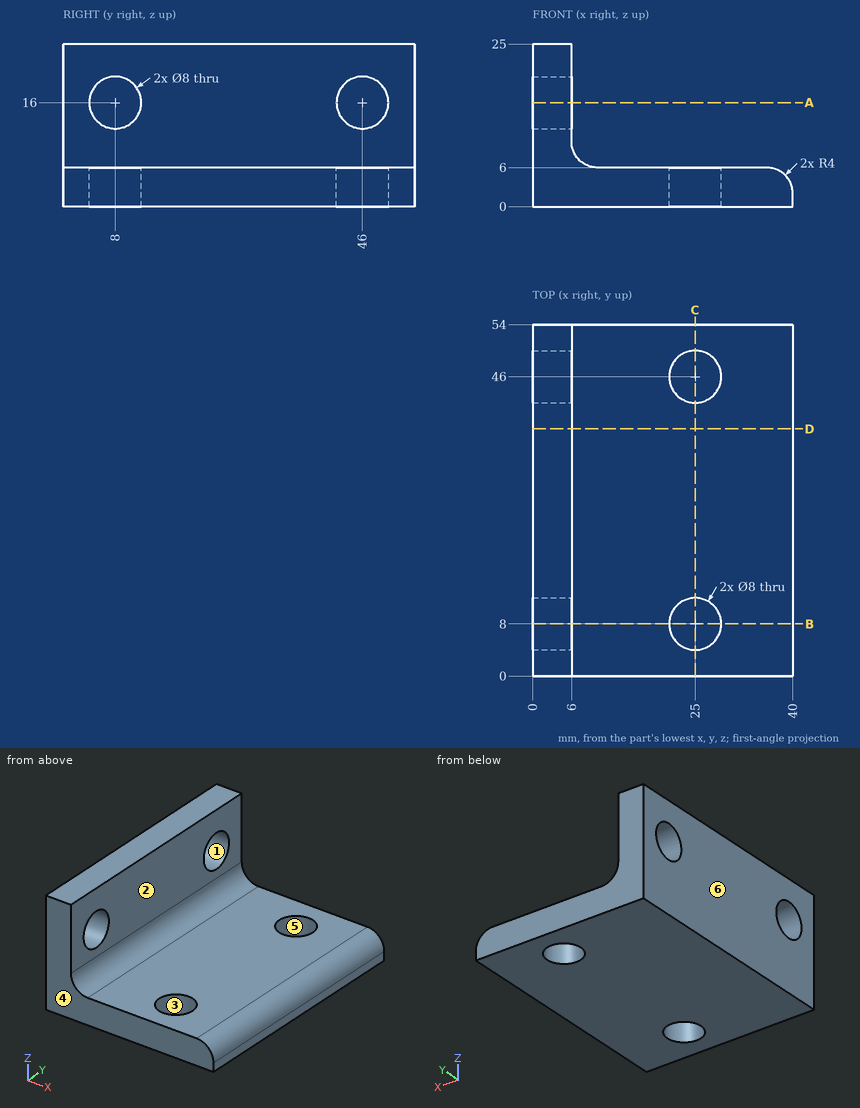
Input: dimensioned drawing with shaded views. Units: mm. Origin: part minimum x, y, z. A direction names the side the tool comes from. Give positions to 0.01 mm unless a question says otherwise; leave off trailing zeros. Write each loop counter-clockwise with the first axis right and the second up, starting at its lowest first coordinate (ties: lowest second). Pieces come first, ordered by that corner, then holes. Notation, with made-up numbers: (62.5, -27) - (92.5, -27) arc R23 ccw to (92.5, -15) - close; hole circle Ø4 at (-12.5, 86). An arc over 180 degrees is marked (long way). Write item = value, one per line. Start each with the question number.
1) Cut plane A-A (z = 16). Return loops of the section in (x, y), and give its area (3 significant figures).
2) Cut plane C-C (x = 25). Return loops of the section in (y, z), and give its area (3 significant figures).
3) Material intervals for L1, parallel to X at y = 8, z = 2.1; L2, parallel to Y at x = 2, z = 12.5; L3, parallel to Z at x = 1.7, y = 46, sorted ascending. Write a range as [from, to].
4) Pin query (flat end, axial travel): pin 1 (4 mm diameter, centred on x = 23.5, y = 16, fed in from -Z); pin 2 (7.5 mm diameter, centred on y = 23, z = 21, fed in from +X); pin 3 (6 mm diameter, centred on x = 30, y = 23.5, fed in from +Z). Return the tip coordinate at first contact, or that it passes through.
5) Reachability of the marked faces 1 and 2 from +Z, -Z, +X, -X, +Y, -Y: full face, straight path, thin tool, end or side. Return the list, or none.
6) Draft query along X for the marked faces 3, 4, 5 and 6. Return one class per face: pulls with the +X half, pulls with the -X half, needs draft (parallel to the pull), parting line crosses it, or undercut.
7) Cut plane D-D (y = 38). Return loops of the section in (x, z).
8) Cut plane B-B (y = 8). Return loops of the section in (x, z).
Answers follow:
q1.outline = (0, 0) - (6, 0) - (6, 4) - (0, 4) - close; (0, 12) - (6, 12) - (6, 42) - (0, 42) - close; (0, 50) - (6, 50) - (6, 54) - (0, 54) - close
q1.area = 228 mm^2
q2.outline = (0, 0) - (4, 0) - (4, 6) - (0, 6) - close; (12, 0) - (42, 0) - (42, 6) - (12, 6) - close; (50, 0) - (54, 0) - (54, 6) - (50, 6) - close
q2.area = 228 mm^2
q3.L1 = [0, 21], [29, 40]
q3.L2 = [0, 6.06], [9.94, 44.06], [47.94, 54]
q3.L3 = [0, 12], [20, 25]
q4.pin_1 = 0
q4.pin_2 = 6
q4.pin_3 = 6
q5.face_1 = +X, -X
q5.face_2 = +Z, +X, +Y, -Y
q6.face_3 = undercut
q6.face_4 = needs draft
q6.face_5 = undercut
q6.face_6 = pulls with the -X half
q7.outline = (0, 0) - (40, 0) - (40, 2) arc R4 ccw to (36, 6) - (10, 6) arc R4 cw to (6, 10) - (6, 25) - (0, 25) - close
q8.outline = (0, 0) - (21, 0) - (21, 6) - (10, 6) arc R4 cw to (6, 10) - (6, 12) - (0, 12) - close; (0, 20) - (6, 20) - (6, 25) - (0, 25) - close; (29, 0) - (40, 0) - (40, 2) arc R4 ccw to (36, 6) - (29, 6) - close
